Geometry: see drawing. Coordinates: mm, zero at the bounding-box minimum. A direction names the side the tool comes from. Coordinates: 2 decimals unless noted, no trailing zeros. Answer as a JSON object with one key per item and string values. Group by question number.
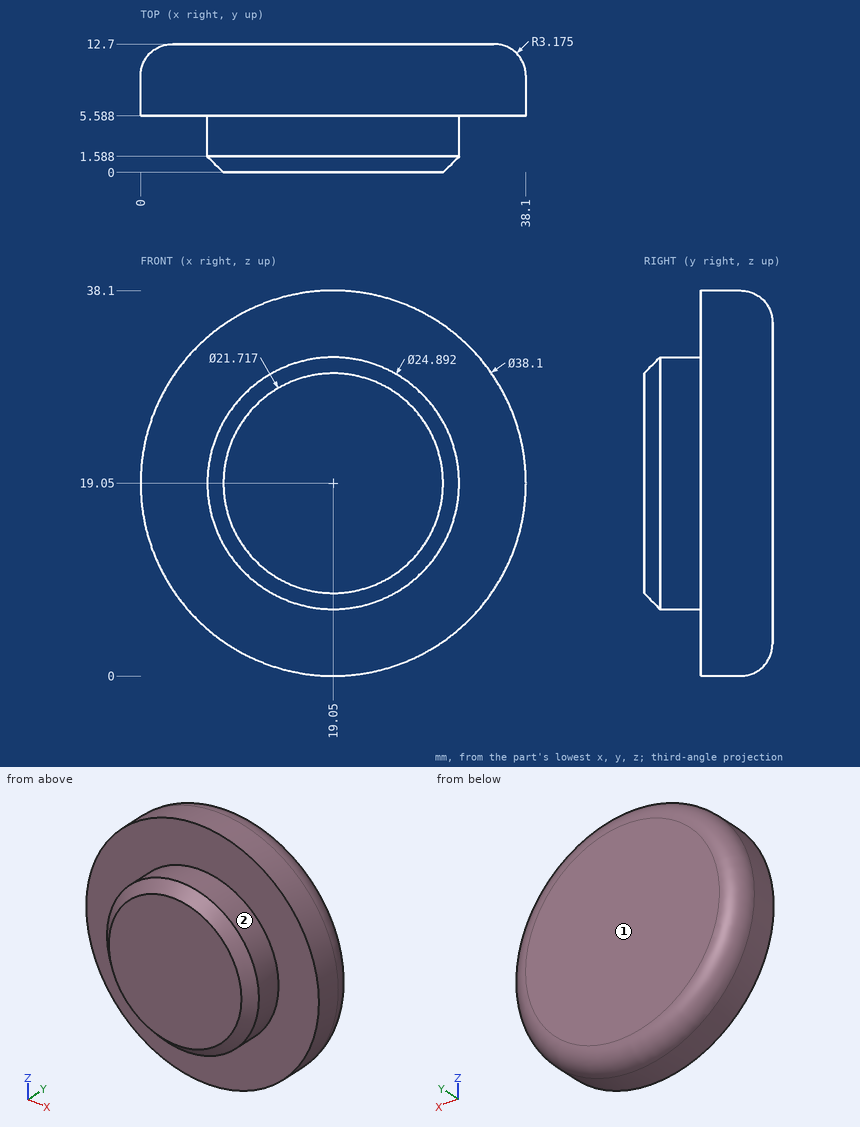
Item 1: Contact query for flat-ended pins moving along their axis: pin 1 (5 mm diameter, centred on x = 17.5, y = 6, fed in from -Z); pin 2 (1.5 mm diameter, centred on y = 10.5, z = 9, fed in from -X); pin 3 (3 mm diameter, centred on x = 25, y = 5.5, fed in from -Z). Output: stop coordinate, or through.
Item 2: Set-up query: the marked faces 1 and 2. Return all of +Z, -Z, +X, -X, +Y, -Y with unobstructed straight access to the full face (end or side cutting, diameter ignored); none if empty.
Item 3: Ray query, L1, parallel to Y at x = 16.5, z = 32; L2, parallel to Z at x = 28, y = 4; L3, parallel to Z at x = 6, y = 7.5. Return the intervals inside material, ascending. Write a range as [from, to].
Answer sheet:
{
 "1": {"pin 1": "stops at z = 0", "pin 2": "stops at x = 2.54", "pin 3": "stops at z = 0.53"},
 "2": {"face 1": "+Z, -Z, +X, -X, +Y", "face 2": "-Y"},
 "3": {"L1": "y = [5.59, 12.7]", "L2": "z = [10.4, 27.7]", "L3": "z = [5.17, 32.93]"}
}
